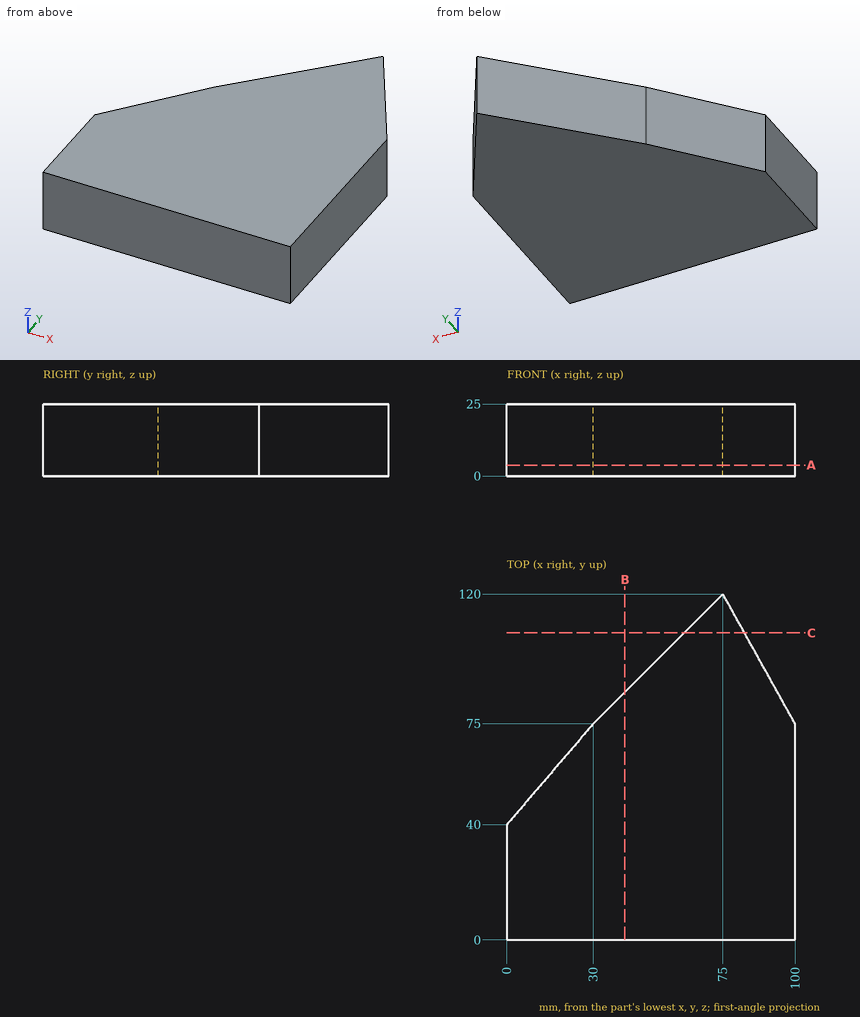
Geometry check sheet. Reference: drawing and pictorial views, mm from the part's lowest x, y, z. Coordinates: 2 decimals unless noted, no trailing zeros. Order: outer loops, then holes, each group sorted by start corner. A loop starts at its lowest first (then second) coordinate and runs counter-clockwise, first axis right, second up. Notation, with made-up numbers: (-22, 50.5) - (-6, 50.5) arc R21 cw to (-6, 70.5) - close; hole circle Ø3 at (76.5, 41.5). An arc over 180 degrees is marked (long way). One line per item, written item: value.
(1) Depth check by flat-ended pin: pin 1 Ø4 at (y, z) = (76.5, 12) entering from -X; pin 2 Ø3 at (x, z) = (23, 16) entering from +Y. Enter the tip coordinate at first touch or a pass-through.
Data:
pin 1: stops at x = 29.57
pin 2: stops at y = 68.58
(2) Sectioned sample at A-A (z = 3.75). Enter the section's corners in (x, y), and give its area (3 significant figures).
Data:
outline: (0, 0) - (100, 0) - (100, 75) - (75, 120) - (30, 75) - (0, 40) - close
area: 8,550 mm^2
(3) Thickness scan on probe 1 along Y at (x, z) = (55, 6); probe 2 along X at (y, z) = (52, 9.25); probe 3 along Y at (x, z) = (80.5, 6.75). Record the ranges inside material, lowest first. Write a range as from..to.
Data:
probe 1: y = 0..100
probe 2: x = 10.29..100
probe 3: y = 0..110.1
(4) Sectioned sample at B-B (x = 41). Enter the section's corners in (y, z).
Data:
outline: (0, 0) - (86, 0) - (86, 25) - (0, 25) - close
(5) Sectioned sample at C-C (y = 106.5). Enter the section's corners in (x, z).
Data:
outline: (61.5, 0) - (82.5, 0) - (82.5, 25) - (61.5, 25) - close
